```python
from build123d import *

# Parameters (mm, degrees)
F0_W     = 11
F0_H     = 30
F1_DEPTH = 24
F3_DEPTH = 11
F4_R     = 5
F4_R_2   = 2.5
F5_DEPTH = 41.001
F6_R     = 13
F7_R     = 5
F8_R     = 2


# Not quite as in the source:
# - ends of sketch curves that miss each other by under 0.0002 mm in the source are joined


with BuildPart() as f1:
    # F0 (on Right) → F1 (new body, symmetric)
    with BuildSketch(Plane.YZ):
        with BuildLine():
            Line((-56, 0), (-30, 0))
            ThreePointArc((-30, 0), (-29.4730143031, 5.5983415304), (-27.9105714739, 11))
            Line((-27.9105714739, 11), (-56, 11))
            Line((-56, 11), (-56, 0))
        make_face()
        with BuildLine():
            Line((-30, 0), (-19, 0))
            ThreePointArc((-19, 0), (-18.1017503893, 5.7729223833), (-15.4919333848, 11))
            Line((-15.4919333848, 11), (-27.9105714739, 11))
            ThreePointArc((-27.9105714739, 11), (-29.4730143031, 5.5983415304), (-30, 0))
        make_face()
        with BuildLine():
            ThreePointArc((-15.4919333848, 11), (0, 19), (15.4919333848, 11))
            Line((15.4919333848, 11), (27.9105714739, 11))
            ThreePointArc((27.9105714739, 11), (0, 30), (-27.9105714739, 11))
            Line((-27.9105714739, 11), (-15.4919333848, 11))
        make_face()
        with BuildLine():
            ThreePointArc((15.4919333848, 11), (18.1017503893, 5.7729223833), (19, 0))
            Line((19, 0), (30, 0))
            ThreePointArc((30, 0), (29.4730143031, 5.5983415304), (27.9105714739, 11))
            Line((27.9105714739, 11), (15.4919333848, 11))
        make_face()
        with BuildLine():
            ThreePointArc((27.9105714739, 11), (29.4730143031, 5.5983415304), (30, 0))
            Line((30, 0), (51, 0))
            Line((51, 0), (51, 11))
            Line((51, 11), (40, 11))
            Line((40, 11), (27.9105714739, 11))
        make_face()
        with Locations((45.5, 26)):
            Rectangle(F0_W, F0_H)
    extrude(amount=F1_DEPTH, both=True)

    # F2 (on face) → F3 (cut, through all)
    with BuildSketch(Plane(origin=(0, 51, 0), x_dir=(-1, 0, 0), z_dir=(0, 1, 0))):
        with BuildLine():
            Line((-6.4943742253, 25.2703764435), (-6.4943742253, 24.7296235565))
            ThreePointArc((-6.4943742253, 24.7296235565), (0.1340750741, 18.501382926), (6.4999995983, 24.9977146924))
            ThreePointArc((6.4999995983, 24.9977146924), (6.4999998996, 24.9988573462), (6.5, 25))
            ThreePointArc((6.5, 25), (0.1352174827, 31.4985934041), (-6.4943742253, 25.2703764435))
        make_face()
        with BuildLine():
            Line((-6.4943742253, 41), (-6.4943742253, 25.2703764435))
            ThreePointArc((-6.4943742253, 25.2703764435), (0.1352174827, 31.4985934041), (6.5, 25))
            Line((6.5, 25), (6.5056257747, 41))
            Line((6.5056257747, 41), (-6.4943742253, 41))
        make_face()
    extrude(amount=-F3_DEPTH, mode=Mode.SUBTRACT)

    # F4 (on Top) → F5 (cut, through all)
    with BuildSketch(Plane.XY):
        with Locations((11, -42.9459065199)):
            Circle(F4_R)
        with Locations((-11, -42.9459065199)):
            Circle(F4_R)
        Circle(F4_R_2)
    extrude(amount=F5_DEPTH, mode=Mode.SUBTRACT)

    # F6
    f6_edges = [f1.edges().sort_by_distance(p)[0] for p in [
        (-24, -56, 5.5),
        (24, -56, 5.5),
    ]]
    fillet(f6_edges, radius=F6_R)

    # F7
    f7_edges = [f1.edges().sort_by_distance(p)[0] for p in [
        (-24, 45.5, 41),
        (24, 45.5, 41),
    ]]
    fillet(f7_edges, radius=F7_R)

    # F8
    f8_edges = [f1.edges().sort_by_distance(p)[0] for p in [
        (0, -27.910571, 11),
        (0, 27.910571, 11),
    ]]
    fillet(f8_edges, radius=F8_R)


solid = f1.part
```
Could you check a few things on this model? Use its own coordinates, in mm. A direction names the side the tool comes from. Give positions to 0.01 mm unless a question says otherwise; leave off trailing zeros. Loops run counter-clockwise (first coordinate to the right, second up) from the corner with the lowest first, then second, coordinate; pieces in that order, holes last. Notation, with made-up numbers: (86.5, -9) -> (130.5, -9) arc R23 cw to (130.5, 9) -> close; hole circle Ø4 at (58.5, 87). An arc over 180 degrees is marked (long way). Put each result on its own line as item: value.
(1) For faces 1 (the face through (0, 35, 11)), 2 (the face through (6.494, 46, 33)), 3 (the face through (23, 46, 39)), which set-ups out of +Z, -Z, +X, -X, +Y, -Y let a thin tool reach every point of the face, with its end or its side?
Computed:
face 1: +Z, +X, -X
face 2: +Z, +Y
face 3: +Z, +X, +Y, -Y
(2) Imagine slicing it at C-C on x = 0. Write out the boundary of the cut face in (y, z), plus the area to 3 significant figures.
Computed:
outline: (-56, 0) -> (-19, 0) arc R19 cw to (-2.5, 18.83) -> (-2.5, 29.9) arc R30 ccw to (-27.41, 12.19) arc R2 cw to (-29.24, 11) -> (-56, 11) -> close; (2.5, 18.83) arc R19 cw to (19, 0) -> (51, 0) -> (51, 18.5) -> (40, 18.5) -> (40, 11) -> (29.24, 11) arc R2 cw to (27.41, 12.19) arc R30 ccw to (2.5, 29.9) -> close
area: 1,410 mm^2
(3) I'm going to push flat-ended pins straight in: pin 1 Ø1 at (x, z) = (13, 10) entering from -Y; pin 2 Ø15 at (x, z) = (9, 27.5) entering from -Y; pin 3 Ø13 at (x, y) = (-11, -42.95) entering from -Z; pin 4 Ø1 at (x, y) = (16.5, 2.5) entering from +Z. Where does each tip first touch, or does it pass through?
Computed:
pin 1: y = -55.91
pin 2: y = -22.36
pin 3: z = 0
pin 4: z = 29.93
(4) Imagine slicing it at D-D on z = 37.5. Write out the boundary of the cut face in (x, y), plus the area to 3 significant figures.
Computed:
outline: (-23.77, 40) -> (-6.5, 40) -> (-6.5, 51) -> (-23.77, 51) -> close; (6.49, 40) -> (23.77, 40) -> (23.77, 51) -> (6.49, 51) -> close
area: 380 mm^2
(5) Thinking about a two-plate mould opening in X: for faces 4 (the face through (-20.293, -52.091, 5.423)), 5 (the face through (-13, 45, 41)), 6 (the face through (-8.69, -47.38, 5.42)), which applies, pulls with the +X half, pulls with the -X half, needs draft (parallel to the pull), parting line crosses it, or undercut?
Computed:
face 4: pulls with the -X half
face 5: needs draft
face 6: undercut
(6) Please list where these lines run through material, in increasing order: probe 1 along Y at (x, z) = (-11.5, 8); probe 2 along Z at (x, y) = (22, 38); probe 3 along Y at (x, z) = (5, 8). Write a range as [from, to].
Computed:
probe 1: [-55.99, -47.92], [-37.97, -17.23], [17.23, 51]
probe 2: [0, 11]
probe 3: [-56, -17.23], [17.23, 51]
(7) Imagine slicing it at A-A on z = 3.5. Write out the boundary of the cut face in (x, y), plus the area to 3 significant figures.
Computed:
outline: (-24, -43) arc R13 ccw to (-11, -56) -> (11, -56) arc R13 ccw to (24, -43) -> (24, -18.67) -> (-24, -18.67) -> close; (-24, 18.67) -> (24, 18.67) -> (24, 51) -> (-24, 51) -> close; hole circle Ø10 at (-11, -42.95); hole circle Ø10 at (11, -42.95)
area: 3,110 mm^2
(8) Imagine slicing it at B-B on y = 1.5. Write out the boundary of the cut face in (x, z), plus the area to 3 significant figures.
Computed:
outline: (-24, 18.94) -> (-2, 18.94) -> (-2, 29.96) -> (-24, 29.96) -> close; (2, 18.94) -> (24, 18.94) -> (24, 29.96) -> (2, 29.96) -> close
area: 485 mm^2
